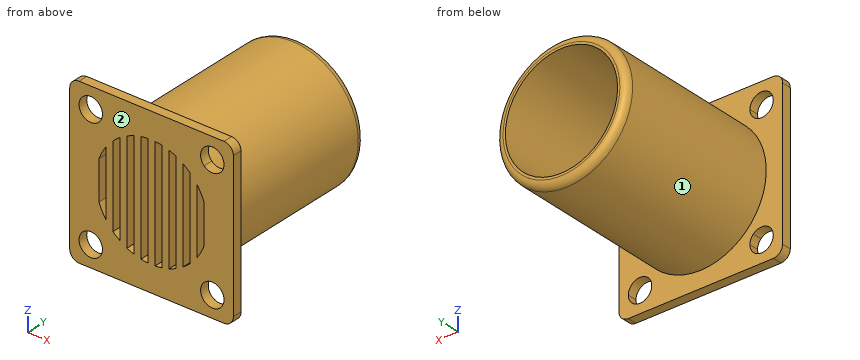
from build123d import *
from build123d.topology import SkipClean

# Parameters (mm, degrees)
ESBO_O1_W                = 35
ESBO_O1_H                = 35
RESSALTO_EXTRUS_O1_DEPTH = 2
FILETE2_R                = 2
ESBO_O3_R                = 14
ESBO_O3_R_2              = 12
RESSALTO_EXTRUS_O3_DEPTH = 36.5
FILETE3_R                = 1.5


with BuildPart() as part:
    # Esboço1 → Ressalto-extrusão1 (new body)
    with BuildSketch(Plane(origin=(0, 0, 0), x_dir=(1, 0, 0), z_dir=(0, 1, 0))):
        Rectangle(ESBO_O1_W, ESBO_O1_H)
        with BuildLine():
            ThreePointArc((-10.5, -13), (-15.304886114, -13.968245837), (-11.25, -11.214642893))
            ThreePointArc((-11.25, -11.214642893), (-10.695113886, -12.031754163), (-10.5, -13))
        make_face(mode=Mode.SUBTRACT)
        with BuildLine():
            ThreePointArc((15.5, -13), (12.031754163, -15.304886114), (11.25, -11.214642893))
            ThreePointArc((11.25, -11.214642893), (13.968245837, -10.695113886), (15.5, -13))
        make_face(mode=Mode.SUBTRACT)
        with BuildLine():
            ThreePointArc((-9.75, -6.99553429), (-10.59422921, -5.635805838), (-11.25, -4.175823272))
            Line((-11.25, -4.175823272), (-11.25, 4.175823272))
            ThreePointArc((-11.25, 4.175823272), (-10.59422921, 5.635805838), (-9.75, 6.99553429))
            Line((-9.75, 6.99553429), (-9.75, -6.99553429))
        make_face(mode=Mode.SUBTRACT)
        with BuildLine():
            ThreePointArc((-6.75, -9.921567416), (-7.524255874, -9.348025115), (-8.25, -8.714212529))
            Line((-8.25, -8.714212529), (-8.25, 8.714212529))
            ThreePointArc((-8.25, 8.714212529), (-7.524255874, 9.348025115), (-6.75, 9.921567416))
            Line((-6.75, 9.921567416), (-6.75, -9.921567416))
        make_face(mode=Mode.SUBTRACT)
        with BuildLine():
            ThreePointArc((-3.75, -11.399013115), (-4.510269977, -11.120137802), (-5.25, -10.790620927))
            Line((-5.25, -10.790620927), (-5.25, 10.790620927))
            ThreePointArc((-5.25, 10.790620927), (-4.510269977, 11.120137802), (-3.75, 11.399013115))
            Line((-3.75, 11.399013115), (-3.75, -11.399013115))
        make_face(mode=Mode.SUBTRACT)
        with BuildLine():
            Line((-0.75, 11.976539567), (-0.75, -11.976539567))
            ThreePointArc((-0.75, -11.976539567), (-1.502985267, -11.905504411), (-2.25, -11.787175234))
            Line((-2.25, -11.787175234), (-2.25, 11.787175234))
            ThreePointArc((-2.25, 11.787175234), (-1.502985267, 11.905504411), (-0.75, 11.976539567))
        make_face(mode=Mode.SUBTRACT)
        with BuildLine():
            ThreePointArc((-10.5, 13), (-10.695113886, 12.031754163), (-11.25, 11.214642893))
            ThreePointArc((-11.25, 11.214642893), (-15.304886114, 13.968245837), (-10.5, 13))
        make_face(mode=Mode.SUBTRACT)
        with BuildLine():
            ThreePointArc((2.25, -11.787175234), (1.502985267, -11.905504411), (0.75, -11.976539567))
            Line((0.75, -11.976539567), (0.75, 11.976539567))
            ThreePointArc((0.75, 11.976539567), (1.502985267, 11.905504411), (2.25, 11.787175234))
            Line((2.25, 11.787175234), (2.25, -11.787175234))
        make_face(mode=Mode.SUBTRACT)
        with BuildLine():
            ThreePointArc((5.25, -10.790620927), (4.510269977, -11.120137802), (3.75, -11.399013115))
            Line((3.75, -11.399013115), (3.75, 11.399013115))
            ThreePointArc((3.75, 11.399013115), (4.510269977, 11.120137802), (5.25, 10.790620927))
            Line((5.25, 10.790620927), (5.25, -10.790620927))
        make_face(mode=Mode.SUBTRACT)
        with BuildLine():
            ThreePointArc((8.25, -8.714212529), (7.524255874, -9.348025115), (6.75, -9.921567416))
            Line((6.75, -9.921567416), (6.75, 9.921567416))
            ThreePointArc((6.75, 9.921567416), (7.524255874, 9.348025115), (8.25, 8.714212529))
            Line((8.25, 8.714212529), (8.25, -8.714212529))
        make_face(mode=Mode.SUBTRACT)
        with BuildLine():
            ThreePointArc((11.25, -4.175823272), (10.59422921, -5.635805838), (9.75, -6.99553429))
            Line((9.75, -6.99553429), (9.75, 6.99553429))
            ThreePointArc((9.75, 6.99553429), (10.59422921, 5.635805838), (11.25, 4.175823272))
            Line((11.25, 4.175823272), (11.25, -4.175823272))
        make_face(mode=Mode.SUBTRACT)
        with BuildLine():
            ThreePointArc((15.5, 13), (13.968245837, 10.695113886), (11.25, 11.214642893))
            ThreePointArc((11.25, 11.214642893), (12.031754163, 15.304886114), (15.5, 13))
        make_face(mode=Mode.SUBTRACT)
    extrude(amount=RESSALTO_EXTRUS_O1_DEPTH)

    # Filete2
    filete2_edges = [part.edges().sort_by_distance(p)[0] for p in [
        (-17.5, 1, 17.5),
        (-17.5, 1, -17.5),
        (17.5, 1, -17.5),
        (17.5, 1, 17.5),
    ]]
    fillet(filete2_edges, radius=FILETE2_R)

    # Esboço3 → Ressalto-extrusão3 (add)
    with SkipClean():  # the faces are left unmerged after this step: merging them gives an invalid solid
        with BuildSketch(Plane(origin=(0, 2, 0), x_dir=(1, 0, 0), z_dir=(0, 1, 0))):
            with Locations(Location((0, 0, 0), (0, 0, 270))):
                Circle(ESBO_O3_R)
            with Locations(Location((0, 0, 0), (0, 0, 86.416678302))):
                Circle(ESBO_O3_R_2, mode=Mode.SUBTRACT)
        extrude(amount=RESSALTO_EXTRUS_O3_DEPTH)

    # Filete3
    filete3_edges = [part.edges().sort_by_distance(p)[0] for p in [
        (0, 38.5, -14),
    ]]
    fillet(filete3_edges, radius=FILETE3_R)


solid = part.part
The listing builds one solid part. Answer for the finished solid, in the listing's coordinates (mm). Face numbers are marked on the shaded views. A direction names the side the tool comes from. Round coordinates to 2 decimals unless told otherwise and drop trailing zeros. Order: outer loops, then holes, each group sorted by start corner. A loop starts at its lowest first (then second) coordinate and runs counter-clockwise, first axis right, second up. Notation, with made-up numbers: (5, -37.5) -> (13, -37.5) arc R34 ccw to (13, -4.5) -> close; hole circle Ø9 at (36, -31). An arc over 180 degrees is marked (long way). One line per item, written item: value.
Item 1: Find section B-B, the plane y = 13. Give the vertices of the cut face in (x, z).
Taken from the geometry:
outline: circle Ø28 at (0, 0); hole circle Ø24 at (0, 0)
Item 2: Find section A-A, the plane z = 0. State how many separate pieces and enclosed holes the cut face has, then the cut area to 3 significant figures.
Taken from the geometry:
separate pieces: 9
enclosed holes: 0
area: 191 mm2
Item 3: Given P1, Ø10, axis at x = -2, y = 9, coming from the +Z side; P2, Ø8, axis at x = 0, z = 2, coming from the -Y side; P3, Ø1.7, axis at x = -9, z = -4.5, coming from the +Y side; P4, Ø12, axis at x = -4, y = 16, coming from the -Z side, each flat-ended and moving along its own axis, determine where each tip first touches the part or whether it passes through.
Taken from the geometry:
P1: stops at z = 14
P2: stops at y = 0
P3: stops at y = 2
P4: stops at z = -14
Item 4: For the marked faces 1 and 2, determine the directions among +Z, -Z, +X, -X, +Y, -Y from which every point of the face is accessible in a straight line to the end or side of a thin tool.
Taken from the geometry:
face 1: +Y
face 2: +Z, -Z, +X, -X, -Y
Item 5: Straight lines are drawn through the part: L1, parallel to Z at x = -13, y = 0.7; L2, parallel to X at y = 18.5, z = 0. For each, find the intervals that lie inside material, in ascending order.
Taken from the geometry:
L1: z = -17.5 to -15.5, -10.5 to 10.5, 15.5 to 17.5
L2: x = -14 to -12, 12 to 14
